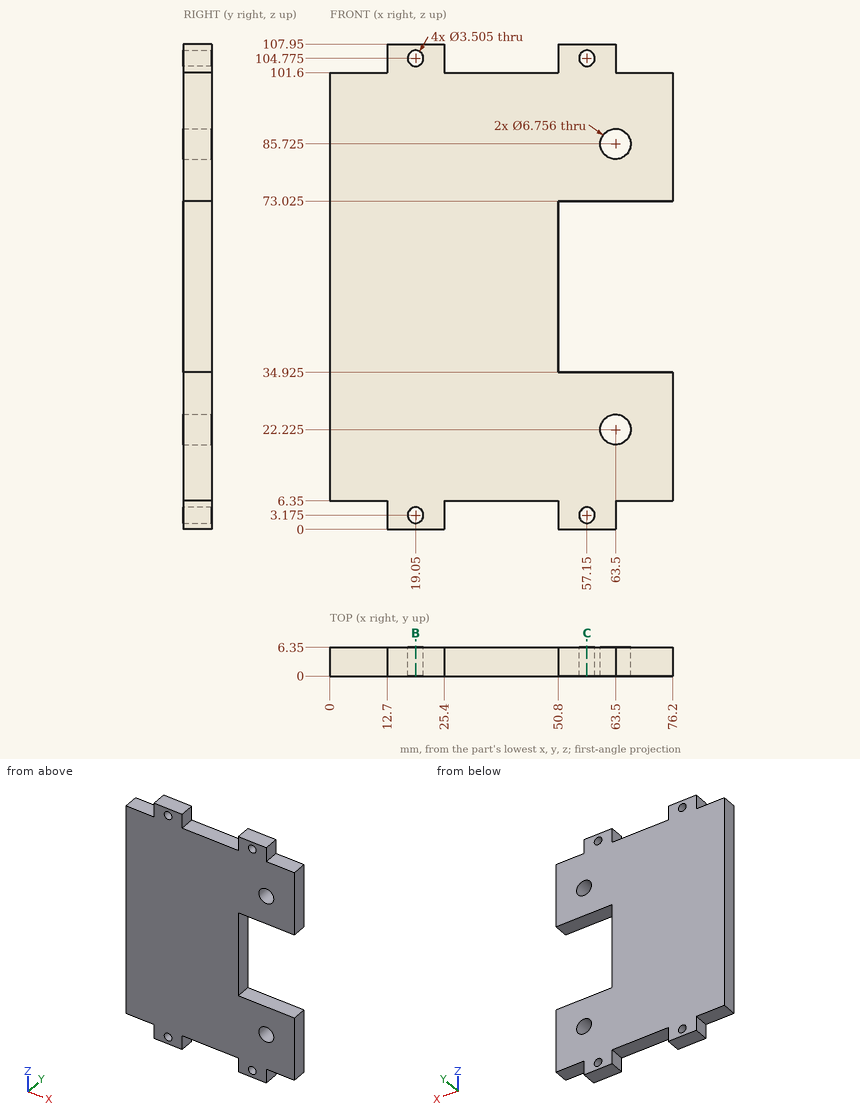
Check sheet for the drawn part. Datum: minimum x, y, z corner. Units: mm. Round coordinates to 2 decimals unless told otherwise and drop trailing zeros. Write each loop counter-clockwise with the first axis right and the second up, starting at its lowest first coordinate (ties: lowest second). Pieces come first, ordered by that corner, then holes. Notation, with made-up numbers: (8, -21.75) - (48, -21.75) arc R6 cw to (48, -17.75) - close; hole circle Ø5 at (6, 87). An arc over 180 degrees is marked (long way). Write each question's results on one line, items separated by ' | '.
(1) Depth check by flat-ended pin: pin 1 Ø3 at (x, z) = (57.15, 3.175) entering from -Y; pin 2 Ø1.9 at (x, y) = (5.5, 4.5) entering from +Z; pin 3 Ø1.9 at (x, y) = (9.5, 2) entering from -Z; pin 4 Ø1.9 at (y, z) = (2.5, 103.5) entering from +X. Enter the tip coordinate at first touch or a pass-through.
Computed:
pin 1: passes through | pin 2: stops at z = 101.6 | pin 3: stops at z = 6.35 | pin 4: stops at x = 63.5
(2) Thickness scan on probe 1 along X at (y, z) = (2.5, 50); probe 2 along Z at (x, y) = (31.5, 2.5); probe 3 along X at (y, z) = (2.5, 86.5). Record the ranges inside material, lowest first. Write a range as from..to.
Computed:
probe 1: x = 0..50.8 | probe 2: z = 6.35..101.6 | probe 3: x = 0..60.21, 66.79..76.2
(3) Sectioned sample at C-C, the plane x = 57.15. Count the separate pieces of the cut face and the enclosed holes in it, plus the area to 3 significant figures.
Computed:
separate pieces: 4 | enclosed holes: 0 | area: 399 mm^2
(4) Sectioned sample at B-B, the plane x = 19.05. Enter the section's corners in (y, z).
Computed:
outline: (0, 0) - (6.35, 0) - (6.35, 1.42) - (0, 1.42) - close; (0, 4.93) - (6.35, 4.93) - (6.35, 103.02) - (0, 103.02) - close; (0, 106.53) - (6.35, 106.53) - (6.35, 107.95) - (0, 107.95) - close
